Geometry: final body of the model. Coordinates: model frame, mm. A direction names the side the tool comes from. Round coordinates to 2 decimals unless told otherwise and drop trailing zeros. Loops run counter-clockwise (first coordinate to the right, second up) from the corner with the lowest first, then second, coordinate; pieces in that order, holes last. Notation, with made-up numbers: M 75,58 L 88,58 A16 ccw 88,89 Z; hole C -33.75,28 d5. An arc over 180 degrees is marked long. Answer as a JSON object with one key per item and string values.
from build123d import *

# Parameters (mm, degrees)
BOSS_EXTRUDE1_DEPTH = 5.1
SKETCH2_R           = 2.1
BOSS_EXTRUDE2_DEPTH = 0.9
FILLET1_R           = 2
SKETCH3_R           = 2.1
BOSS_EXTRUDE3_DEPTH = 1.1
BOSS_EXTRUDE4_DEPTH = 16.158031


with BuildPart() as part:
    # Sketch1 → Boss-Extrude1 (new body)
    with BuildSketch(Plane.XY):
        with BuildLine():
            Line((99.95, 149.85), (25.05, 149.85))
            Line((25.05, 149.85), (25.05, 148))
            Line((25.05, 148), (25.05, 111.5))
            ThreePointArc((25.05, 111.5), (25.591852455, 110.191852455), (26.9, 109.65))
            Line((26.9, 109.65), (98.1, 109.65))
            ThreePointArc((98.1, 109.65), (99.408147545, 110.191852455), (99.95, 111.5))
            Line((99.95, 111.5), (99.95, 148))
            Line((99.95, 148), (99.95, 149.85))
        make_face()
    extrude(amount=BOSS_EXTRUDE1_DEPTH)

    # Sketch2 → Boss-Extrude2 (add)
    with BuildSketch(Plane.XY.offset(5.1)):
        with BuildLine():
            Line((102.1, 149.85), (22.9, 149.85))
            Line((22.9, 149.85), (9.05, 149.85))
            Line((9.05, 149.85), (9.05, 148))
            Line((9.05, 148), (9.05, 143.30803115))
            ThreePointArc((9.05, 143.30803115), (9.351726371, 142.295436082), (10.158485157, 141.61314008))
            Line((10.158485157, 141.61314008), (23.761760493, 135.66170712))
            ThreePointArc((23.761760493, 135.66170712), (24.699345028, 134.868768523), (25.05, 133.69196885))
            Line((25.05, 133.69196885), (25.05, 111.5))
            ThreePointArc((25.05, 111.5), (25.591852455, 110.191852455), (26.9, 109.65))
            Line((26.9, 109.65), (98.1, 109.65))
            ThreePointArc((98.1, 109.65), (99.408147545, 110.191852455), (99.95, 111.5))
            Line((99.95, 111.5), (99.95, 133.69196885))
            ThreePointArc((99.95, 133.69196885), (100.300654972, 134.868768523), (101.238239507, 135.66170712))
            Line((101.238239507, 135.66170712), (114.841514843, 141.61314008))
            ThreePointArc((114.841514843, 141.61314008), (115.648273629, 142.295436082), (115.95, 143.30803115))
            Line((115.95, 143.30803115), (115.95, 148))
            Line((115.95, 148), (115.95, 149.85))
            Line((115.95, 149.85), (102.1, 149.85))
        make_face()
        with Locations((16.3, 145.05)):
            Circle(SKETCH2_R, mode=Mode.SUBTRACT)
        with Locations((108.7, 145.05)):
            Circle(SKETCH2_R, mode=Mode.SUBTRACT)
    extrude(amount=BOSS_EXTRUDE2_DEPTH)

    # Fillet1
    fillet1_edges = [part.edges().sort_by_distance(p)[0] for p in [
        (25.05, 149.85, 2.55),
        (99.95, 149.85, 2.55),
        (115.95, 149.85, 5.55),
        (9.05, 149.85, 5.55),
    ]]
    fillet(fillet1_edges, radius=FILLET1_R)

    # Sketch3 → Boss-Extrude3 (add)
    with BuildSketch(Plane.XY.offset(6)):
        with BuildLine():
            Line((99.95, 133.69196885), (99.95, 149.85))
            Line((99.95, 149.85), (113.95, 149.85))
            ThreePointArc((113.95, 149.85), (115.364213562, 149.264213562), (115.95, 147.85))
            Line((115.95, 147.85), (115.95, 143.30803115))
            ThreePointArc((115.95, 143.30803115), (115.648273629, 142.295436082), (114.841514843, 141.61314008))
            Line((114.841514843, 141.61314008), (101.238239507, 135.66170712))
            ThreePointArc((101.238239507, 135.66170712), (100.300654972, 134.868768523), (99.95, 133.69196885))
        make_face()
        with Locations((108.7, 145.05)):
            Circle(SKETCH3_R, mode=Mode.SUBTRACT)
        with BuildLine():
            Line((11.05, 149.85), (25.05, 149.85))
            Line((25.05, 149.85), (25.05, 133.69196885))
            ThreePointArc((25.05, 133.69196885), (24.699345028, 134.868768523), (23.761760493, 135.66170712))
            Line((23.761760493, 135.66170712), (10.158485157, 141.61314008))
            ThreePointArc((10.158485157, 141.61314008), (9.351726371, 142.295436082), (9.05, 143.30803115))
            Line((9.05, 143.30803115), (9.05, 147.85))
            ThreePointArc((9.05, 147.85), (9.635786438, 149.264213562), (11.05, 149.85))
        make_face()
        with Locations((16.3, 145.05)):
            Circle(SKETCH3_R, mode=Mode.SUBTRACT)
    extrude(amount=BOSS_EXTRUDE3_DEPTH)

    # Sketch4 → Boss-Extrude4 (add)
    with BuildSketch(Plane(origin=(0, 149.85, 0), x_dir=(1, 0, 0), z_dir=(0, 1, 0))):
        Polygon((25.05, -7.1), (27.55, -6), (25.05, -6), align=None)
        Polygon((97.45, -6), (99.95, -7.1), (99.95, -6), align=None)
    extrude(amount=-BOSS_EXTRUDE4_DEPTH)


solid = part.part
1) Section query D-D (y = 119). Return the cut outline in (x, z).
Results:
{"outline": "M 25.05,0 L 99.95,0 L 99.95,6 L 25.05,6 Z"}
2) Section query C-C (z = 3.75). Return the cut outline in (x, y).
Results:
{"outline": "M 25.05,111.5 A1.85 ccw 26.9,109.65 L 98.1,109.65 A1.85 ccw 99.95,111.5 L 99.95,147.85 A2 ccw 97.95,149.85 L 27.05,149.85 A2 ccw 25.05,147.85 Z"}
3) Reachability of faces 1 (the flat face through (26.28, 141.88, 6.56)), 2 (the cylindrical face through (25.62, 149.25, 2.59)), 3 (the flat face through (106, 144, 7.1)) from +Z, -Z, +X, -X, +Y, -Y: full face, straight path, thin tool, end or side. Return the list, or none.
Results:
{"face 1": "+Z, +Y, -Y", "face 2": "-Z, -X, +Y", "face 3": "+Z, +X, -X, +Y, -Y"}
4) Pin query (flat end, axial travel): P1, Ø1.5, axis at y = 123.5, z = 2, coming from the +X side; P2, Ø2, axis at y = 140, z = 5, coming from the -X side; P3, Ø6.5, axis at x = 16.3, y = 145.05, coming from the -Z side. Return the tip coordinate at first contact, or that it passes through.
Results:
{"P1": "x = 99.95", "P2": "x = 11.57", "P3": "z = 5.1"}
5) Section query B-B (x = 16.3). Return the cut outline in (y, z), and give its area (3 significant figures).
Results:
{"outline": "M 138.93,5.1 L 142.95,5.1 L 142.95,7.1 L 138.93,7.1 Z; M 147.15,5.1 L 149.85,5.1 L 149.85,7.1 L 147.15,7.1 Z", "area": "13.4 mm2"}
6) Ray query, line 1 (X direction, y = 145.05, z = 5.9); line 2 (X direction, y = 145.05, z = 6.3); line 3 (Z direction, x = 37.5, y = 119). Return the intervals inside material, ascending.
Results:
{"line 1": "9.05 to 14.2, 18.4 to 106.6, 110.8 to 115.95", "line 2": "9.05 to 14.2, 18.4 to 26.87, 98.13 to 106.6, 110.8 to 115.95", "line 3": "0 to 6"}
7) Section query A-A (y = 145.05). Return the cut outline in (x, z), and give its area (3 significant figures).
Results:
{"outline": "M 9.05,5.1 L 14.2,5.1 L 14.2,7.1 L 9.05,7.1 Z; M 18.4,5.1 L 25.05,5.1 L 25.05,0 L 99.95,0 L 99.95,5.1 L 106.6,5.1 L 106.6,7.1 L 99.95,7.1 L 97.45,6 L 27.55,6 L 25.05,7.1 L 18.4,7.1 Z; M 110.8,5.1 L 115.95,5.1 L 115.95,7.1 L 110.8,7.1 Z", "area": "499 mm2"}
